Build history of the part. All positions in model axes, mm. Face numbers are marked on the shaded views. A direction names the side the tool comes from. Round coordinates to 2 decimals unless told otherwise and drop trailing zeros. Write each loop counter-clockwise with the first axis right and the second up, starting at its lowest first coordinate (ties: lowest second). Pieces come first, ordered by that corner, then holes. Notation, with made-up numbers: M 64,-32.5 L 81,-32.5 A22 cw 81,-11.5 Z; hole C -23,-11.75 d8. An arc over 180 degrees is marked long. Write item = value, one per line. Start each with the question number.
Q1. Band-saw the part on C-C on x = 7. Write the cut outline in (y, z).
Q2. Probe L1, parallel to Y at x = -11, z = 25; L2, parallel to X at y = 62, z = 0; L3, parallel to Z at x = -7, y = 56. List the from-to ranges inside material, lowest first.
Q3. Band-saw the part on D-D on y = 20. Write the cut outline in (x, z).
Q4. Tool access for the marked faces 5, 6 and 7: list every direction of +Z, -Z, +X, -X, +Y, -Y with a clear straight run to the whole face (end or side of a thin tool).
Q5. Band-saw the part on A-A on y = 53. State how many separate pieces and enclosed holes the cut face has, plus the area to 3 significant figures.
Q6. Drop flat-ended pins along their axis: P1, Ø4, axis at x = -6, z = 29, coming from the -Y side; P2, Ø4, axis at y = 53, z = 25, coming from the +X side; P3, Ø1.5, axis at x = 7, z = 6.5, coming from the +Y side; P4, Ø3, axis at y = 19, z = 24, coming from the +X side. Give the stop position or say it passes through.
Q7. Pull direction Y, two halves, no side cores. Call the marked faces 1, 2, 3 and 4: released by +Y, released by -Y, zero draft, split by the parting line, or undercut.
```python
from build123d import *

# Parameters (mm, degrees)
SKETCH1_W           = 19
SKETCH1_H           = 17
SKETCH1_R           = 6.1
BOSS_EXTRUDE1_DEPTH = 68
SKETCH3_W           = 65
SKETCH3_H           = 30
CUT_EXTRUDE1_DEPTH  = 17
SKETCH4_W           = 5
SKETCH4_H           = 4
BOSS_EXTRUDE2_DEPTH = 3
SKETCH5_W           = 30
SKETCH5_H           = 10
BOSS_EXTRUDE3_DEPTH = 20
SKETCH6_R           = 3.5
CUT_EXTRUDE2_DEPTH  = 59
SKETCH8_R           = 2.1
CUT_EXTRUDE3_DEPTH  = 48.5
SKETCH9_W           = 3.5
SKETCH9_H           = 7
CUT_EXTRUDE4_DEPTH  = 43


with BuildPart() as part:
    # Sketch1 → Boss-Extrude1 (new body)
    with BuildSketch(Plane(origin=(0, 0, 0), x_dir=(1, 0, 0), z_dir=(0, 1, 0))):
        with Locations((-23, 0.5)):
            Rectangle(SKETCH1_W, SKETCH1_H)
        with Locations((-23, 0)):
            Circle(SKETCH1_R, mode=Mode.SUBTRACT)
        with Locations((23, 0.5)):
            Rectangle(SKETCH1_W, SKETCH1_H)
        with Locations((23, 0)):
            Circle(SKETCH1_R, mode=Mode.SUBTRACT)
        Polygon((-13.5, -8), (13.5, -8), (32.5, -8), (32.5, -13), (-32.5, -13), (-32.5, -8), align=None)
    extrude(amount=BOSS_EXTRUDE1_DEPTH)

    # Sketch3 → Cut-Extrude1 (cut)
    with BuildSketch(Plane(origin=(0, 0, -9), x_dir=(-1, 0, 0), z_dir=(0, 0, -1))):
        with Locations((0, 34)):
            Rectangle(SKETCH3_W, SKETCH3_H)
    extrude(amount=-CUT_EXTRUDE1_DEPTH, mode=Mode.SUBTRACT)

    # Sketch4 → Boss-Extrude2 (add)
    with BuildSketch(Plane(origin=(0, 0, 8), x_dir=(-1, 0, 0), z_dir=(0, 0, -1))):
        with BuildLine():
            ThreePointArc((4.191236083, 59.518146972), (4.82097308, 63.804174702), (1.17903595, 66.15))
            Line((1.17903595, 66.15), (-8.82096405, 66.15))
            Line((-8.82096405, 66.15), (-8.82096405, 62.15))
            Line((-8.82096405, 62.15), (1.17903595, 62.15))
            ThreePointArc((1.17903595, 62.15), (3.230210626, 61.45792056), (4.191236083, 59.518146972))
        make_face()
        with Locations((-6.32096405, 56.15)):
            Rectangle(SKETCH4_W, SKETCH4_H)
    extrude(amount=BOSS_EXTRUDE2_DEPTH)

    # Sketch5 → Boss-Extrude3 (add)
    with BuildSketch(Plane.XY.offset(13)):
        with Locations((0, 20)):
            Rectangle(SKETCH5_W, SKETCH5_H)
        with Locations((0, 53)):
            Rectangle(SKETCH5_W, SKETCH5_H)
    extrude(amount=BOSS_EXTRUDE3_DEPTH)

    # Sketch6 → Cut-Extrude2 (cut, through all)
    with BuildSketch(Plane(origin=(0, 58, 0), x_dir=(1, 0, 0), z_dir=(0, 1, 0))):
        with Locations((0, -25)):
            Circle(SKETCH6_R)
    extrude(amount=-CUT_EXTRUDE2_DEPTH, mode=Mode.SUBTRACT)

    # Sketch8 → Cut-Extrude3 (cut, through all)
    with BuildSketch(Plane.ZY.offset(15)):
        with Locations((25, 20)):
            Circle(SKETCH8_R)
        with Locations((25, 53)):
            Circle(SKETCH8_R)
    extrude(amount=-CUT_EXTRUDE3_DEPTH, mode=Mode.SUBTRACT)

    # Sketch9 → Cut-Extrude4 (cut)
    with BuildSketch(Plane.XZ.offset(-15)):
        with Locations((-8.25, 25)):
            Rectangle(SKETCH9_W, SKETCH9_H)
    extrude(amount=-CUT_EXTRUDE4_DEPTH, mode=Mode.SUBTRACT)


solid = part.part
```
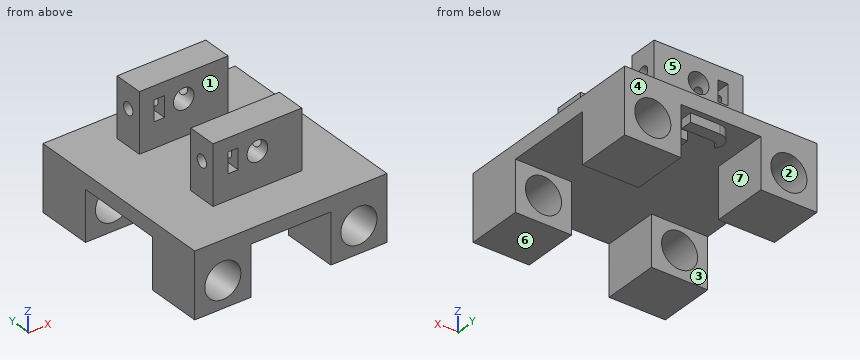
Conclusion:
q1.outline = M 0,8 L 54.15,8 L 54.15,5 L 58.15,5 L 58.15,8 L 62.15,8 L 62.15,5 L 66.15,5 L 66.15,8 L 68,8 L 68,13 L 58,13 L 58,33 L 48,33 L 48,13 L 25,13 L 25,33 L 15,33 L 15,13 L 0,13 Z; hole C 20,25 d4.2; hole C 53,25 d4.2
q2.L1 = 15 to 17.9, 22.1 to 25, 48 to 50.9, 55.1 to 58
q2.L2 = -32.5 to -29.1, -16.9 to -13.5, 13.5 to 16.9, 29.1 to 32.5
q2.L3 = 8 to 21.5, 28.5 to 33
q3.outline = M -32.5,8 L 32.5,8 L 32.5,13 L 15,13 L 15,22.9 L 2.8,22.9 A3.5 cw -2.8,22.9 L -6.5,22.9 L -6.5,21.5 L -10,21.5 L -10,22.9 L -15,22.9 L -15,13 L -32.5,13 Z; M -15,27.1 L -10,27.1 L -10,28.5 L -6.5,28.5 L -6.5,27.1 L -2.8,27.1 A3.5 cw 2.8,27.1 L 15,27.1 L 15,33 L -15,33 Z
q4.face_5 = +Z, +X, -X, +Y
q4.face_6 = -Z, +X, -X, +Y, -Y
q4.face_7 = -Z, +Y, -Y
q5.separate_pieces = 2
q5.enclosed_holes = 2
q5.area = 1,190 mm^2
q6.P1 = 15
q6.P2 = through
q6.P3 = 66.15
q6.P4 = 15
q7.face_1 = undercut
q7.face_2 = zero draft
q7.face_3 = undercut
q7.face_4 = released by +Y
